Work out the finished part from the listing and answer in its coordinate system (mm). A direction names the side the tool comes from. Give positions to 0.01 mm unless a question says otherwise; leave off trailing zeros. Order: outer loops, then holes, each group sorted by start corner. A loop starts at its lowest first (then second) coordinate and runs counter-clockwise, first axis right, second up. Notation, with made-up numbers: M -4.5,10 L 18.5,10 A12 cw 18.5,18 Z; hole C -25,43.25 d5. An arc over 180 degrees is marked long. One line per item, written item: value.
from build123d import *

# Parameters (mm, degrees)
F0_R     = 16.75
F0_R_2   = 1.5
F0_R_3   = 6
F1_DEPTH = 25
F0_R_4   = 21.5
F2_DEPTH = 2


with BuildPart() as f1:
    # F0 (on Right) → F1 (new body)
    with BuildSketch(Plane.YZ):
        Circle(F0_R)
        with Locations((0, -10)):
            Circle(F0_R_2, mode=Mode.SUBTRACT)
        with Locations((-10, 0)):
            Circle(F0_R_2, mode=Mode.SUBTRACT)
        Circle(F0_R_3, mode=Mode.SUBTRACT)
        with Locations((10, 0)):
            Circle(F0_R_2, mode=Mode.SUBTRACT)
        with Locations((0, 10)):
            Circle(F0_R_2, mode=Mode.SUBTRACT)
    extrude(amount=F1_DEPTH)

    # F0 (on Right) → F2 (join)
    with BuildSketch(Plane.YZ):
        Circle(F0_R_4)
        Circle(F0_R, mode=Mode.SUBTRACT)
        Circle(F0_R)
        with Locations((0, -10)):
            Circle(F0_R_2, mode=Mode.SUBTRACT)
        with Locations((-10, 0)):
            Circle(F0_R_2, mode=Mode.SUBTRACT)
        Circle(F0_R_3, mode=Mode.SUBTRACT)
        with Locations((10, 0)):
            Circle(F0_R_2, mode=Mode.SUBTRACT)
        with Locations((0, 10)):
            Circle(F0_R_2, mode=Mode.SUBTRACT)
    extrude(amount=-F2_DEPTH)


solid = f1.part
(1) Find the intervals of material crossed by probe 1 along X at (y, z) = (-14, 16); probe 2 along Y at (x, z) = (14, -1); probe 3 along Z at (x, y) = (11.75, -10), in increasing order. Write a range as from..to.
Findings:
probe 1: x = -2..0
probe 2: y = -16.72..-11.12, -8.88..-5.92, 5.92..8.88, 11.12..16.72
probe 3: z = -13.44..-1.5, 1.5..13.44
(2) Section B-B, the plane x = 10.25 is taken. Give the vertices of the cut face in (y, z).
Findings:
outline: C 0,0 d33.5; hole C -10,0 d3; hole C 0,0 d12; hole C 0,-10 d3; hole C 0,10 d3; hole C 10,0 d3
(3) Section D-D, the plane y = -5 is taken. Give the vertices of the cut face in (x, z).
Findings:
outline: M -2,-20.91 L 0,-20.91 L 0,-15.99 L 25,-15.99 L 25,-3.32 L -2,-3.32 Z; M -2,3.32 L 25,3.32 L 25,15.99 L 0,15.99 L 0,20.91 L -2,20.91 Z
(4) Section A-A, the plane y = 0 is taken. Give the vertices of the cut face in (x, z).
Findings:
outline: M -2,-21.5 L 0,-21.5 L 0,-16.75 L 25,-16.75 L 25,-11.5 L -2,-11.5 Z; M -2,-8.5 L 25,-8.5 L 25,-6 L -2,-6 Z; M -2,6 L 25,6 L 25,8.5 L -2,8.5 Z; M -2,11.5 L 25,11.5 L 25,16.75 L 0,16.75 L 0,21.5 L -2,21.5 Z
(5) Given P1, Ø5, axis at y = 10, z = 0, coming from the -X side; P2, Ø1.5, axis at x = 3.5, z = 15.5, coming from the -Y side; P3, Ø2, axis at x = 15, z = -14, coming from the +Y side; P4, Ø3, axis at x = 11, y = -16.5, coming from the +Z side, each flat-ended and moving along its own axis, determine where each tip first touches the part or whether it passes through.
Findings:
P1: stops at x = -2
P2: stops at y = -7.94
P3: stops at y = 10.56
P4: stops at z = 7.45
(6) Section C-C, the plane z = -10 is taken. Give the vertices of the cut face in (x, y).
Findings:
outline: M -2,-19.03 L 0,-19.03 L 0,-13.44 L 25,-13.44 L 25,-1.5 L -2,-1.5 Z; M -2,1.5 L 25,1.5 L 25,13.44 L 0,13.44 L 0,19.03 L -2,19.03 Z
(7) Which of the six approach directions +Z, -Z, +X, -X, +Y, -Y give full straight-line access (tool end or side, diameter ignored) to faces 1 (the cylindrical face through (-0.986, -2.799, 21.317)), 2 (the flat face through (0, 11, -13))?
Findings:
face 1: +X, -X
face 2: +X
